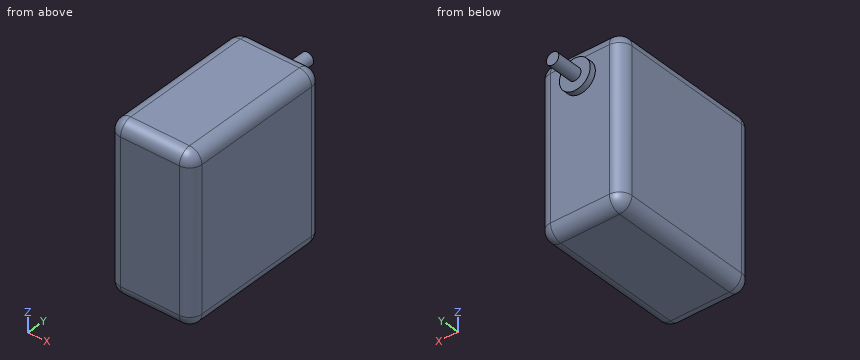
```python
from build123d import *

# Parameters (mm, degrees)
F0_W     = 20.32
F0_H     = 40.64
F0_R     = 3.75
F0_R_2   = 1.499247
F1_DEPTH = 38.1
F2_DEPTH = 1.5
F3_R     = 3
F4_DEPTH = 8


with BuildPart() as f1:
    # F0 (on Front) → F1 (new body)
    with BuildSketch(Plane.XZ):
        Rectangle(F0_W, F0_H)
        with Locations((0, 12.952523)):
            Circle(F0_R, mode=Mode.SUBTRACT)
        with Locations((0, 12.952523)):
            Circle(F0_R)
        with Locations((0, 12.952523)):
            Circle(F0_R_2, mode=Mode.SUBTRACT)
        with Locations((0, 12.952523)):
            Circle(F0_R_2)
    extrude(amount=F1_DEPTH)

    # F0 (on Front) → F2 (join)
    with BuildSketch(Plane.XZ):
        with Locations((0, 12.952523)):
            Circle(F0_R)
        with Locations((0, 12.952523)):
            Circle(F0_R_2, mode=Mode.SUBTRACT)
    extrude(amount=-F2_DEPTH)

    # F3
    f3_edges = [f1.edges().sort_by_distance(p)[0] for p in [
        (10.16, -19.05, -20.32),
        (10.16, -19.05, 20.32),
        (10.16, 0, 0),
        (10.16, -38.1, 0),
        (-10.16, -19.05, 20.32),
        (0, 0, 20.32),
        (0, -38.1, 20.32),
        (-10.16, -19.05, -20.32),
        (-10.16, 0, 0),
        (-10.16, -38.1, 0),
        (0, -38.1, -20.32),
        (0, 0, -20.32),
    ]]
    fillet(f3_edges, radius=F3_R)

    # F0 (on Front) → F4 (join)
    with BuildSketch(Plane.XZ):
        with Locations((0, 12.952523)):
            Circle(F0_R_2)
    extrude(amount=-F4_DEPTH)


solid = f1.part
```
Part model, mm, in its own coordinate system. Round coordinates to 2 decimals unless told otherwise and drop trailing zeros. Loops run counter-clockwise (first coordinate to the right, second up) from the corner with the lowest first, then second, coordinate; pieces in that order, holes last.
Item 1: Cut at B-B, the plane z = 5. Give the cut face in (x, y).
Item 2: Cut at A-A, the plane x = 0. Give the cut face in (y, z), then the cut area to 3 significant figures.
Item 3: Cut at C-C, the plane x = 6.25. Give the cut face in (y, z).
Item 4: Drop a flat-ended pin along its axis: P1, Ø8, axis at x = -2.5, z = -12, coming from the +Y side. Give the stop position or say it passes through.
Item 5: Drill centre lines: line 1 (Y direction, x = 2.5, z = 5); line 2 (Y direction, x = -3.5, z = 14); line 3 (X direction, y = -3, z = 17.5). Where is each one in solid material? Low to high.
A:
1. outline: (-10.16, -35.1) arc R3 ccw to (-7.16, -38.1) - (7.16, -38.1) arc R3 ccw to (10.16, -35.1) - (10.16, -3) arc R3 ccw to (7.16, 0) - (-7.16, 0) arc R3 ccw to (-10.16, -3) - close
2. outline: (-38.1, -17.32) arc R3 ccw to (-35.1, -20.32) - (-3, -20.32) arc R3 ccw to (0, -17.32) - (0, 9.2) - (1.5, 9.2) - (1.5, 11.45) - (8, 11.45) - (8, 14.45) - (1.5, 14.45) - (1.5, 16.7) - (0, 16.7) - (0, 17.32) arc R3 ccw to (-3, 20.32) - (-35.1, 20.32) arc R3 ccw to (-38.1, 17.32) - close
2. area: 1,570 mm2
3. outline: (-38.1, -17.32) arc R3 ccw to (-35.1, -20.32) - (-3, -20.32) arc R3 ccw to (0, -17.32) - (0, 17.32) arc R3 ccw to (-3, 20.32) - (-35.1, 20.32) arc R3 ccw to (-38.1, 17.32) - close
4. P1: stops at y = 0
5. line 1: y = -38.1 to 0
5. line 2: y = -38.1 to 1.5
5. line 3: x = -10.15 to 10.15
